from build123d import *

# Parameters (mm, degrees)
F0_R     = 37
F1_DEPTH = 4


with BuildPart() as f1:
    # F0 (on Top) → F1 (new body)
    with BuildSketch(Plane.XY):
        with Locations((-0.6144908867, -20.3631758839)):
            Circle(F0_R)
        with BuildLine():
            ThreePointArc((-3.1126967397, 12.5421271465), (-0.6618478689, 15.1363755392), (1.8855091133, 12.6368241161))
            ThreePointArc((1.8855091133, 12.6368241161), (1.8850605363, 12.589467134), (1.8837149663, 12.5421271464))
            ThreePointArc((1.8837149663, 12.5421271465), (5.2227863742, 12.1164514875), (8.5011233102, 11.3528386484))
            ThreePointArc((8.5011233102, 11.3528386484), (18.7824224389, 6.3343849305), (26.7323517041, -1.8929241175))
            ThreePointArc((26.7323517041, -1.8929241175), (28.4716524971, -4.7748384787), (29.9083239169, -7.8189430869))
            ThreePointArc((29.9083239169, -7.8189430869), (32.2012610114, -8.1155997543), (33.270374151, -10.1656150695))
            ThreePointArc((33.270374151, -10.1656150695), (32.7647179948, -11.6731271366), (31.4523000449, -12.570812998))
            ThreePointArc((31.4523000449, -12.570812998), (32.0792882461, -15.8779996316), (32.3661111061, -19.2318526816))
            ThreePointArc((32.3661111061, -19.2318526816), (32.3806592551, -19.7974311378), (32.3855091133, -20.3631758839))
            ThreePointArc((32.3855091133, -20.3631758839), (30.5909369208, -31.0972932369), (25.4024015163, -40.6639470438))
            ThreePointArc((25.4024015163, -40.6639470438), (23.199011587, -43.2086809107), (20.7478519472, -45.5157166828))
            ThreePointArc((20.7478519472, -45.5157166828), (21.1450029953, -46.2432936637), (21.2824224389, -47.0607366982))
            ThreePointArc((21.2824224389, -47.0607366982), (19.5097871405, -49.4525854792), (16.7056699662, -48.452533798))
            ThreePointArc((16.7056699662, -48.452533798), (13.7540985771, -50.0708118857), (10.6530279173, -51.3799942249))
            ThreePointArc((10.6530279173, -51.3799942249), (-0.6144908867, -53.3631758839), (-11.8820096908, -51.3799942249))
            ThreePointArc((-11.8820096908, -51.3799942249), (-14.9830803506, -50.0708118857), (-17.9346517396, -48.452533798))
            ThreePointArc((-17.9346517396, -48.452533798), (-21.4808673431, -49.0832791842), (-21.9768337207, -45.5157166828))
            ThreePointArc((-21.9768337207, -45.5157166828), (-24.4279933605, -43.2086809107), (-26.6313832898, -40.6639470438))
            ThreePointArc((-26.6313832898, -40.6639470438), (-31.9993559245, -30.5607366982), (-33.5950928796, -19.2318526816))
            ThreePointArc((-33.5950928796, -19.2318526816), (-33.3082700196, -15.8779996316), (-32.6812818184, -12.570812998))
            ThreePointArc((-32.6812818184, -12.570812998), (-34.3769972152, -9.3930725835), (-31.1373056904, -7.8189430869))
            ThreePointArc((-31.1373056904, -7.8189430869), (-29.7006342706, -4.7748384787), (-27.9613334776, -1.8929241175))
            ThreePointArc((-27.9613334776, -1.8929241175), (-20.0114042124, 6.3343849305), (-9.7301050837, 11.3528386484))
            ThreePointArc((-9.7301050837, 11.3528386484), (-6.4517681477, 12.1164514875), (-3.1126967397, 12.5421271465))
        make_face(mode=Mode.SUBTRACT)
        with BuildLine():
            ThreePointArc((3.5289701119, -17.564652889), (2.3244353747, -16.318090912), (0.7666627795, -15.5577191365))
            Line((0.7666627795, -15.5577191365), (-0.6144908867, -20.3631758839))
            Line((-0.6144908867, -20.3631758839), (3.5289701119, -17.564652889))
        make_face()
        with BuildLine():
            ThreePointArc((0.7666627795, -15.5577191365), (-0.6144908867, -15.3631758839), (-1.9956445529, -15.5577191365))
            Line((-1.9956445529, -15.5577191365), (-0.6144908867, -20.3631758839))
            Line((-0.6144908867, -20.3631758839), (0.7666627795, -15.5577191365))
        make_face()
        with BuildLine():
            Line((-0.6144908867, -20.3631758839), (-1.9956445529, -15.5577191365))
            ThreePointArc((-1.9956445529, -15.5577191365), (-3.5534171482, -16.318090912), (-4.7579518853, -17.564652889))
            Line((-4.7579518853, -17.564652889), (-0.6144908867, -20.3631758839))
        make_face()
        with BuildLine():
            Line((-0.6144908867, -20.3631758839), (-4.7579518853, -17.564652889))
            ThreePointArc((-4.7579518853, -17.564652889), (-5.3697734682, -18.818090912), (-5.6115517947, -20.1917632774))
            Line((-5.6115517947, -20.1917632774), (-0.6144908867, -20.3631758839))
        make_face()
        with BuildLine():
            Line((-4.5564442811, -23.439050302), (-0.6144908867, -20.3631758839))
            Line((-0.6144908867, -20.3631758839), (-5.6115517947, -20.1917632774))
            ThreePointArc((-5.6115517947, -20.1917632774), (-5.3697734682, -21.9082608557), (-4.5564442811, -23.439050302))
        make_face()
        with BuildLine():
            Line((-2.3216907055, -25.0626938143), (-0.6144908867, -20.3631758839))
            Line((-0.6144908867, -20.3631758839), (-4.5564442811, -23.439050302))
            ThreePointArc((-4.5564442811, -23.439050302), (-3.5534171482, -24.4082608557), (-2.3216907055, -25.0626938143))
        make_face()
        with BuildLine():
            Line((1.0927089321, -25.0626938143), (-0.6144908867, -20.3631758839))
            Line((-0.6144908867, -20.3631758839), (-2.3216907055, -25.0626938143))
            ThreePointArc((-2.3216907055, -25.0626938143), (-0.6144908867, -25.3631758839), (1.0927089321, -25.0626938143))
        make_face()
        with BuildLine():
            Line((3.3274625077, -23.439050302), (-0.6144908867, -20.3631758839))
            Line((-0.6144908867, -20.3631758839), (1.0927089321, -25.0626938143))
            ThreePointArc((1.0927089321, -25.0626938143), (2.3244353747, -24.4082608557), (3.3274625077, -23.439050302))
        make_face()
        with BuildLine():
            Line((3.5289701119, -17.564652889), (-0.6144908867, -20.3631758839))
            Line((-0.6144908867, -20.3631758839), (4.3825700213, -20.1917632774))
            ThreePointArc((4.3825700213, -20.1917632774), (4.1407916947, -18.818090912), (3.5289701119, -17.564652889))
        make_face()
        with BuildLine():
            Line((4.3825700213, -20.1917632774), (-0.6144908867, -20.3631758839))
            Line((-0.6144908867, -20.3631758839), (3.3274625077, -23.439050302))
            ThreePointArc((3.3274625077, -23.439050302), (4.1136042356, -21.989557301), (4.3855091133, -20.3631758839))
            ThreePointArc((4.3855091133, -20.3631758839), (4.3847742863, -20.2774569829), (4.3825700213, -20.1917632774))
        make_face()
        with BuildLine():
            ThreePointArc((1.8837149663, 12.5421271464), (-0.6144908867, 10.1368241161), (-3.1126967397, 12.5421271465))
            ThreePointArc((-3.1126967397, 12.5421271465), (-6.4517681477, 12.1164514875), (-9.7301050837, 11.3528386484))
            Line((-9.7301050837, 11.3528386484), (-8.4607071462, 6.9362143197))
            Line((-8.4607071462, 6.9362143197), (-1.9956445529, -15.5577191365))
            ThreePointArc((-1.9956445529, -15.5577191365), (-0.6144908867, -15.3631758839), (0.7666627795, -15.5577191365))
            Line((0.7666627795, -15.5577191365), (7.2317253727, 6.9362143197))
            Line((7.2317253727, 6.9362143197), (8.5011233102, 11.3528386484))
            ThreePointArc((8.5011233102, 11.3528386484), (5.2227863742, 12.1164514875), (1.8837149663, 12.5421271465))
        make_face()
        with BuildLine():
            ThreePointArc((29.9083239169, -7.8189430869), (28.4716524971, -4.7748384787), (26.7323517041, -1.8929241175))
            Line((26.7323517041, -1.8929241175), (22.9241578916, -4.4650052731))
            Line((22.9241578916, -4.4650052731), (3.5289701119, -17.564652889))
            ThreePointArc((3.5289701119, -17.564652889), (4.1407916947, -18.818090912), (4.3825700213, -20.1917632774))
            Line((4.3825700213, -20.1917632774), (32.3661111061, -19.2318526816))
            ThreePointArc((32.3661111061, -19.2318526816), (32.0792882461, -15.8779996316), (31.4523000449, -12.570812998))
            ThreePointArc((31.4523000449, -12.570812998), (28.3927328603, -10.9381575554), (29.9083239169, -7.8189430869))
        make_face()
        with BuildLine():
            ThreePointArc((3.3274625077, -23.439050302), (2.3244353747, -24.4082608557), (1.0927089321, -25.0626938143))
            Line((1.0927089321, -25.0626938143), (10.6530279173, -51.3799942249))
            ThreePointArc((10.6530279173, -51.3799942249), (13.7540985771, -50.0708118857), (16.7056699662, -48.452533798))
            ThreePointArc((16.7056699662, -48.452533798), (17.3129593082, -45.0381942123), (20.7478519472, -45.5157166828))
            ThreePointArc((20.7478519472, -45.5157166828), (23.199011587, -43.2086809107), (25.4024015163, -40.6639470438))
            Line((25.4024015163, -40.6639470438), (21.7794103669, -37.836956291))
            Line((21.7794103669, -37.836956291), (3.3274625077, -23.439050302))
        make_face()
        with BuildLine():
            ThreePointArc((-2.3216907055, -25.0626938143), (-3.5534171482, -24.4082608557), (-4.5564442811, -23.439050302))
            Line((-4.5564442811, -23.439050302), (-26.6313832898, -40.6639470438))
            ThreePointArc((-26.6313832898, -40.6639470438), (-24.4279933605, -43.2086809107), (-21.9768337207, -45.5157166828))
            ThreePointArc((-21.9768337207, -45.5157166828), (-19.1939611779, -44.6981561418), (-17.5114042124, -47.0607366982))
            ThreePointArc((-17.5114042124, -47.0607366982), (-17.6195554314, -47.7881013998), (-17.9346517396, -48.452533798))
            ThreePointArc((-17.9346517396, -48.452533798), (-14.9830803506, -50.0708118857), (-11.8820096908, -51.3799942249))
            Line((-11.8820096908, -51.3799942249), (-10.3129475496, -47.0607366982))
            Line((-10.3129475496, -47.0607366982), (-2.3216907055, -25.0626938143))
        make_face()
        with BuildLine():
            Line((-4.7579518853, -17.564652889), (-27.9613334776, -1.8929241175))
            ThreePointArc((-27.9613334776, -1.8929241175), (-29.7006342706, -4.7748384787), (-31.1373056904, -7.8189430869))
            ThreePointArc((-31.1373056904, -7.8189430869), (-29.9493406093, -8.7347282091), (-29.4993559245, -10.1656150695))
            ThreePointArc((-29.4993559245, -10.1656150695), (-30.4918438573, -12.1599589133), (-32.6812818184, -12.570812998))
            ThreePointArc((-32.6812818184, -12.570812998), (-33.3082700196, -15.8779996316), (-33.5950928796, -19.2318526816))
            Line((-33.5950928796, -19.2318526816), (-29.0023679965, -19.3893954767))
            Line((-29.0023679965, -19.3893954767), (-5.6115517947, -20.1917632774))
            ThreePointArc((-5.6115517947, -20.1917632774), (-5.3697734682, -18.818090912), (-4.7579518853, -17.564652889))
        make_face()
    extrude(amount=F1_DEPTH)


solid = f1.part
CAD build for the part. Positions are in the model's coordinates, mm. A direction names the side the tool comes from. Round coordinates to 2 decimals unless told otherwise and drop trailing zeros. Order: outer loops, then holes, each group sorted by start corner. A loop starts at its lowest first (then second) coordinate and runs counter-clockwise, first axis right, second up. Notation, with made-up numbers: (4.25, -35.5) - (48.25, -35.5) arc R20 ccw to (48.25, -13.5) - close; hole circle Ø4 at (4.5, 11). An arc over 180 degrees is marked (long way). Return JSON: item names as keys, results as strings.
(1) Cut at D-D (z = 3.25). State how many separate pieces and enclosed holes the cut face has, then the cut area to 3 significant figures.
Answer key:
{"separate pieces": "1", "enclosed holes": "10", "area": "2,350 mm^2"}
(2) Pin check, flat tips, straight feed: pin 1 Ø6 at (x, y) = (-8.5, -2) entering from -Z; pin 2 Ø2 at (x, z) = (-22.5, 1) entering from +Y; pin 3 Ø2 at (x, z) = (-5.5, 3.5) entering from +Y; pin 4 Ø1 at (x, z) = (-19.5, 2.5) entering from -Y. Stop position of each tip, or through.
Answer key:
{"pin 1": "stops at z = 0", "pin 2": "stops at y = 10.18", "pin 3": "stops at y = 16.43", "pin 4": "stops at y = -52.47"}
(3) Pull direction Y, two halves, no side cores. Call faces 3 (the face through (-1, -20, 4)), 4 (the face through (-20.14, 6.24, 1.97)), 5 (the face through (-37.58, -18.74, 1.97)): +Y half, -Y half, draft (parallel to the pull), parting line (faces both ways), or undercut.
Answer key:
{"face 3": "draft", "face 4": "undercut", "face 5": "parting line"}
(4) Cut at C-C (y = -3). Give the cut face in (x, z).
Answer key:
{"outline": "(-33.29, 0) - (-26.32, 0) - (-26.32, 4) - (-33.29, 4) - close; (-5.6, 0) - (4.38, 0) - (4.38, 4) - (-5.6, 4) - close; (25.09, 0) - (32.06, 0) - (32.06, 4) - (25.09, 4) - close"}
(5) Tool access for faces 1 (the face through (-1, -20, 0)), 2 (the face through (-31.95, -30.71, 1.97)): list every direction of +Z, -Z, +X, -X, +Y, -Y with a clear straight run to the whole face (end or side of a thin tool).
Answer key:
{"face 1": "-Z, +X, -X, +Y, -Y", "face 2": "+Z, -Z"}
(6) Cut at A-A (y = -29.5). Give the cut face in (x, z) (3 decimals).
Answer key:
{"outline": "(-36.469, 0) - (-32.324, 0) - (-32.324, 4) - (-36.469, 4) - close; (-12.324, 0) - (-3.934, 0) - (-3.934, 4) - (-12.324, 4) - close; (2.705, 0) - (11.095, 0) - (11.095, 4) - (2.705, 4) - close; (31.095, 0) - (35.24, 0) - (35.24, 4) - (31.095, 4) - close"}
(7) Cut at B-B (x = -24). Give the cut face in (y, z), then the cut area to 3 significant figures.
Answer key:
{"outline": "(-49.04, 0) - (-38.61, 0) - (-38.61, 4) - (-49.04, 4) - close; (-19.56, 0) - (-4.57, 0) - (-4.57, 4) - (-19.56, 4) - close; (2.92, 0) - (8.31, 0) - (8.31, 4) - (2.92, 4) - close", "area": "123 mm^2"}
(8) Wall check: probe 1 along X at (y, z) = (-26.5, 2.65); probe 2 along X at (y, z) = (-1.5, 1.3); probe 3 along X at (y, z) = (-6, 1.75). Give the ranges that are in metal, low to high. Write a range as from..to.
Answer key:
{"probe 1": "x = -37.1..-33.04, -8.48..-2.84, 1.61..7.25, 31.81..35.87", "probe 2": "x = -32.44..-27.69, -6.04..4.81, 26.46..31.22", "probe 3": "x = -34.71..-21.88, -4.74..3.51, 20.65..33.48"}
